Could you check a few things on this model? Use its own coordinates, in mm. Face numbers are marked on the shaded views. Give positions to 0.01 mm unless a question says otherwise; leave off trailing zeros. Order: outer loops, then holes, each group sorted by start corner. A loop starts at its lowest first (then second) coordinate and runs counter-clockwise, first axis right, second up.
(1) Imagine slicing it at C-C, the plane z = 0. Write out the boundary of the cut face in (x, y) (3 decimals).
(2) Imagine slicing it at D-D, the plane x = 29.5. Write out the boundary of the cut face in (y, z).
(3) Imagine slicing it at A-A, the plane x = 0. Write out the boundary of the cut face in (y, z) (3 decimals), then the cut area to 3 significant figures.
(4) If we mould it in two halves opening along X, with no side actions, what happens to the marked faces 1, 2 and 3? For each: released by +X, released by -X, zero draft, split by the parting line, or undercut.
(5) Will these pins go through, and if not, where does the flat tip stop? pin 1 (5 mm diameter, centred on y = 1.5, z = -30.5, fed in from -X); pin 2 (2 mm diameter, centred on y = 3.5, z = -15.5, fed in from +X); pin 3 (6 mm diameter, centred on y = 6.35, z = 0, fed in from -X) (3 decimals); pin 4 (1 mm diameter, centred on x = -9.5, y = 8.5, fed in from +Z).
(6) Imagine slicing it at B-B, the plane z = -10. Write out the boundary of the cut face in (x, y).
(7) If I drill on probe 1 along Y at (x, z) = (-39, 0); probe 2 along X at (y, z) = (12.25, 29.5); probe 3 along Z at (x, y) = (3.5, 5.25), over which ranges is the centre line in solid material (lowest first)?
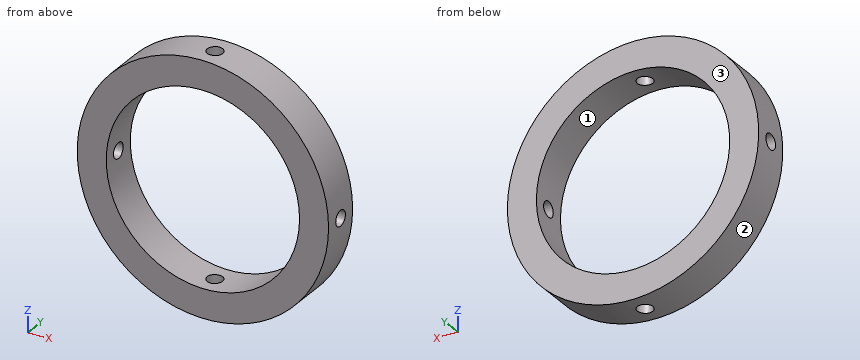
from build123d import *

# Parameters (mm, degrees)
SKETCH1_R           = 41.275
SKETCH1_R_2         = 31.75
BOSS_EXTRUDE1_DEPTH = 12.7
CIRPATTERN1_COUNT   = 4


with BuildPart() as part:
    # Sketch1 → Boss-Extrude1 (new body)
    with BuildSketch(Plane(origin=(0, 0, 0), x_dir=(1, 0, 0), z_dir=(0, 1, 0))):
        Circle(SKETCH1_R)
        Circle(SKETCH1_R_2, mode=Mode.SUBTRACT)
    extrude(amount=BOSS_EXTRUDE1_DEPTH)

    # Sketch3 → #7 (0.201) Diameter Hole1 (revolve, cut)
    with BuildSketch(Plane(origin=(0, 6.35, 41.275), x_dir=(0, -1, 0), z_dir=(1, 0, 0))):
        Polygon((0, 0), (0, 13.217816902), (2.5527, 11.684), (2.5527, 0), align=None)
    f_7_0_201_diameter_hole1 = revolve(axis=Axis((0, 6.35, 47.625), (0, 0, -1)), mode=Mode.SUBTRACT)

    # CirPattern1: #7 (0.201) Diameter Hole1 ×4 about axis
    cirpattern1_axis = Axis((0, -0.3175, 0), (0, 1, 0))
    for i in range(1, CIRPATTERN1_COUNT):
        add(f_7_0_201_diameter_hole1.rotate(cirpattern1_axis, i * 360 / CIRPATTERN1_COUNT), mode=Mode.SUBTRACT)


solid = part.part
Answer block:
1. outline: (-41.275, 0) - (-31.75, 0) - (-31.75, 3.797) - (-41.275, 3.797) - close; (-41.275, 8.903) - (-31.75, 8.903) - (-31.75, 12.7) - (-41.275, 12.7) - close; (31.75, 0) - (41.275, 0) - (41.275, 3.797) - (31.75, 3.797) - close; (31.75, 8.903) - (41.275, 8.903) - (41.275, 12.7) - (31.75, 12.7) - close
2. outline: (0, -28.87) - (12.7, -28.87) - (12.7, -11.74) - (0, -11.74) - close; (0, 11.74) - (12.7, 11.74) - (12.7, 28.87) - (0, 28.87) - close
3. outline: (0, -41.275) - (3.797, -41.275) - (3.797, -31.75) - (0, -31.75) - close; (0, 31.75) - (3.797, 31.75) - (3.797, 41.275) - (0, 41.275) - close; (8.903, -41.275) - (12.7, -41.275) - (12.7, -31.75) - (8.903, -31.75) - close; (8.903, 31.75) - (12.7, 31.75) - (12.7, 41.275) - (8.903, 41.275) - close
3. area: 145 mm2
4. face 1: undercut
4. face 2: split by the parting line
4. face 3: zero draft
5. pin 1: stops at x = -30.33
5. pin 2: stops at x = 38.64
5. pin 3: stops at x = -41.275
5. pin 4: stops at z = 40.28
6. outline: (-40.05, 0) - (-30.13, 0) - (-30.13, 12.7) - (-40.05, 12.7) - close; (30.13, 0) - (40.05, 0) - (40.05, 12.7) - (30.13, 12.7) - close
7. probe 1: y = 0 to 3.8, 8.9 to 12.7
7. probe 2: x = -28.87 to -11.74, 11.74 to 28.87
7. probe 3: z = -41.13 to -31.56, 31.56 to 41.13
